```python
from build123d import *

# Parameters (mm, degrees)
F4_R      = 2.25
F5_DEPTH  = 5
F3_R      = 2
F6_DEPTH  = 5
F2_R      = 1.830021
F7_DEPTH  = 5
F1_R      = 1.5
F8_DEPTH  = 5
F0_R      = 35.5
F9_DEPTH  = 4.5
F11_R     = 1
F12_R     = 4.85
F13_DEPTH = 10
F14_R     = 1


with BuildPart() as f5:
    # F4 (on face) → F5 (new body)
    with BuildSketch(Plane.XY):
        with Locations((0, 30)):
            Circle(F4_R)
        with Locations((-7.764571, 28.977775)):
            Circle(F4_R)
        with Locations((-15, 25.980762)):
            Circle(F4_R)
        with Locations((-21.213203, 21.213203)):
            Circle(F4_R)
        with Locations((-25.980762, 15)):
            Circle(F4_R)
        with Locations((-28.977775, 7.764571)):
            Circle(F4_R)
        with Locations((-30, 0)):
            Circle(F4_R)
        with Locations((-28.977775, -7.764571)):
            Circle(F4_R)
        with Locations((-25.980762, -15)):
            Circle(F4_R)
        with Locations((-21.213203, -21.213203)):
            Circle(F4_R)
        with Locations((-15, -25.980762)):
            Circle(F4_R)
        with Locations((-7.764571, -28.977775)):
            Circle(F4_R)
        with Locations((0, -30)):
            Circle(F4_R)
        with Locations((7.764571, -28.977775)):
            Circle(F4_R)
        with Locations((15, -25.980762)):
            Circle(F4_R)
        with Locations((21.213203, -21.213203)):
            Circle(F4_R)
        with Locations((25.980762, -15)):
            Circle(F4_R)
        with Locations((28.977775, -7.764571)):
            Circle(F4_R)
        with Locations((30, 0)):
            Circle(F4_R)
        with Locations((28.977775, 7.764571)):
            Circle(F4_R)
        with Locations((25.980762, 15)):
            Circle(F4_R)
        with Locations((21.213203, 21.213203)):
            Circle(F4_R)
        with Locations((15, 25.980762)):
            Circle(F4_R)
        with Locations((7.764571, 28.977775)):
            Circle(F4_R)
    extrude(amount=F5_DEPTH)


with BuildPart() as f6:
    # F3 (on face) → F6 (new body)
    with BuildSketch(Plane.XY):
        with Locations((0, 22.5)):
            Circle(F3_R)
        with Locations((-8.610377, 20.787289)):
            Circle(F3_R)
        with Locations((-15.909903, 15.909903)):
            Circle(F3_R)
        with Locations((-20.787289, 8.610377)):
            Circle(F3_R)
        with Locations((-22.5, 0)):
            Circle(F3_R)
        with Locations((-20.787289, -8.610377)):
            Circle(F3_R)
        with Locations((-15.909903, -15.909903)):
            Circle(F3_R)
        with Locations((-8.610377, -20.787289)):
            Circle(F3_R)
        with Locations((0, -22.5)):
            Circle(F3_R)
        with Locations((8.610377, -20.787289)):
            Circle(F3_R)
        with Locations((15.909903, -15.909903)):
            Circle(F3_R)
        with Locations((20.787289, -8.610377)):
            Circle(F3_R)
        with Locations((22.5, 0)):
            Circle(F3_R)
        with Locations((20.787289, 8.610377)):
            Circle(F3_R)
        with Locations((15.909903, 15.909903)):
            Circle(F3_R)
        with Locations((8.610377, 20.787289)):
            Circle(F3_R)
    extrude(amount=F6_DEPTH)


with BuildPart() as f7:
    # F2 (on face) → F7 (new body)
    with BuildSketch(Plane.XY):
        with Locations((0, 15)):
            Circle(F2_R)
        with Locations((-9.641814, 11.490667)):
            Circle(F2_R)
        with Locations((-14.772116, 2.604723)):
            Circle(F2_R)
        with Locations((-12.990381, -7.5)):
            Circle(F2_R)
        with Locations((-5.130302, -14.095389)):
            Circle(F2_R)
        with Locations((5.130302, -14.095389)):
            Circle(F2_R)
        with Locations((12.990381, -7.5)):
            Circle(F2_R)
        with Locations((14.772116, 2.604723)):
            Circle(F2_R)
        with Locations((9.641814, 11.490667)):
            Circle(F2_R)
    extrude(amount=F7_DEPTH)


with BuildPart() as f8:
    # F1 (on face) → F8 (new body)
    with BuildSketch(Plane.XY):
        with Locations((0, 7.5)):
            Circle(F1_R)
        with Locations((-6.495191, 3.75)):
            Circle(F1_R)
        with Locations((-6.495191, -3.75)):
            Circle(F1_R)
        with Locations((0, -7.5)):
            Circle(F1_R)
        with Locations((6.495191, -3.75)):
            Circle(F1_R)
        with Locations((6.495191, 3.75)):
            Circle(F1_R)
    extrude(amount=F8_DEPTH)


with BuildPart() as f9:
    # F0 (on Top) → F9 (new body)
    with BuildSketch(Plane.XY):
        Circle(F0_R)
    extrude(amount=F9_DEPTH)

    # F10: cut F5, F6, F7, F8
    add(f5.part, mode=Mode.SUBTRACT)
    add(f6.part, mode=Mode.SUBTRACT)
    add(f7.part, mode=Mode.SUBTRACT)
    add(f8.part, mode=Mode.SUBTRACT)

    # F11
    f11_edges = [f9.edges().sort_by_distance(p)[0] for p in [
        (-35.5, 0, 0),
        (-35.5, 0, 4.5),
    ]]
    fillet(f11_edges, radius=F11_R)

    # F12 (on face) → F13 (join)
    with BuildSketch(Plane.XY.offset(4.5)):
        Circle(F12_R)
    extrude(amount=F13_DEPTH)

    # F14
    f14_edges = [f9.edges().sort_by_distance(p)[0] for p in [
        (-4.85, 0, 14.5),
    ]]
    fillet(f14_edges, radius=F14_R)


solid = f9.part
```
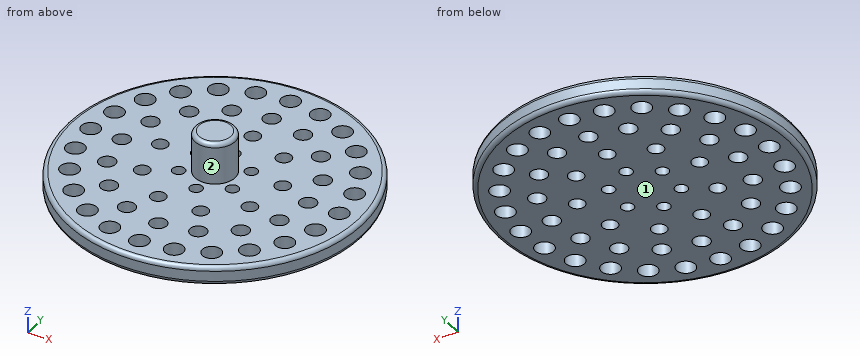
Can you work these out from the model? Positions are in its coordinate system, mm. Face numbers are marked on the shaded views. A direction names the side the tool comes from. Round coordinates to 2 decimals unless told otherwise and drop trailing zeros. Order: outer loops, then holes, each group sorted by start corner. A loop starts at its lowest first (then second) coordinate and runs counter-clockwise, first axis right, second up. Notation, with made-up numbers: (0.25, -32.75) -> (7.25, -32.75) arc R33 cw to (7.25, 0.25) -> close; hole circle Ø10 at (33, -14). An arc over 180 degrees is marked (long way). Return JSON: item names as keys, results as strings. Group by question number.
1. Will these pins go through, and if not, where does the flat tip stop? pin 1 (1.5 mm diameter, centred on x = 3, z = 6.5, fed in from -Y); pin 2 (5 mm diameter, centred on x = 22, y = 22, fed in from +Z); pin 3 (6 mm diameter, centred on x = -4, z = 6.5, fed in from +Y).
2. If we section it at B-B, the plane z = 8: Write out the boundary of the cut face in (x, y).
3. Which directions (+Z, -Z, +X, -X, +Y, -Y) give clear straight access to the entire face, cutting with the end or side of a thin tool? Please do the marked faces 1 and 2.
4. I need wall thicknesses on line 1 (Y direction, x = 22.5, z = 3); line 2 (X direction, y = -3, z = 1.5); line 3 (Z direction, x = 18, y = -13.5). Which ranges of each line are inside material? Lowest first, please. Write a range as [from, to].
5. If we section it at A-A, the plane x = 0: Count the separate pieces of the cut face and the enclosed holes in it, then the cut area to 3 significant figures.
Output values:
{
 "1": {"pin 1": "y = -4.3", "pin 2": "z = 4.5", "pin 3": "y = 35.36"},
 "2": {"outline": "circle Ø9.7 at (0, 0)"},
 "3": {"face 1": "-Z, +X, -X, +Y, -Y", "face 2": "+Z"},
 "4": {"line 1": "[-27.46, -23.06], [-19.37, -9.64], [-7.58, -2], [2, 7.58], [9.64, 19.37], [23.06, 27.46]", "line 2": "[-35.37, -7.79], [-5.2, 5.2], [7.79, 35.37]", "line 3": "[0, 4.5]"},
 "5": {"separate pieces": "8", "enclosed holes": "0", "area": "295 mm²"}
}
